Answer from the drawing. Dimensions are ordinates in mm from the lowest x, y and z of the part. Round coordinates to 2 decimals unless told otherwise and drop trailing zeros. Order: outer loops, then holes, each group sorted by start corner. A loop starts at its lowest first (then second) coordinate and runs counter-clockwise, first axis right, second up.
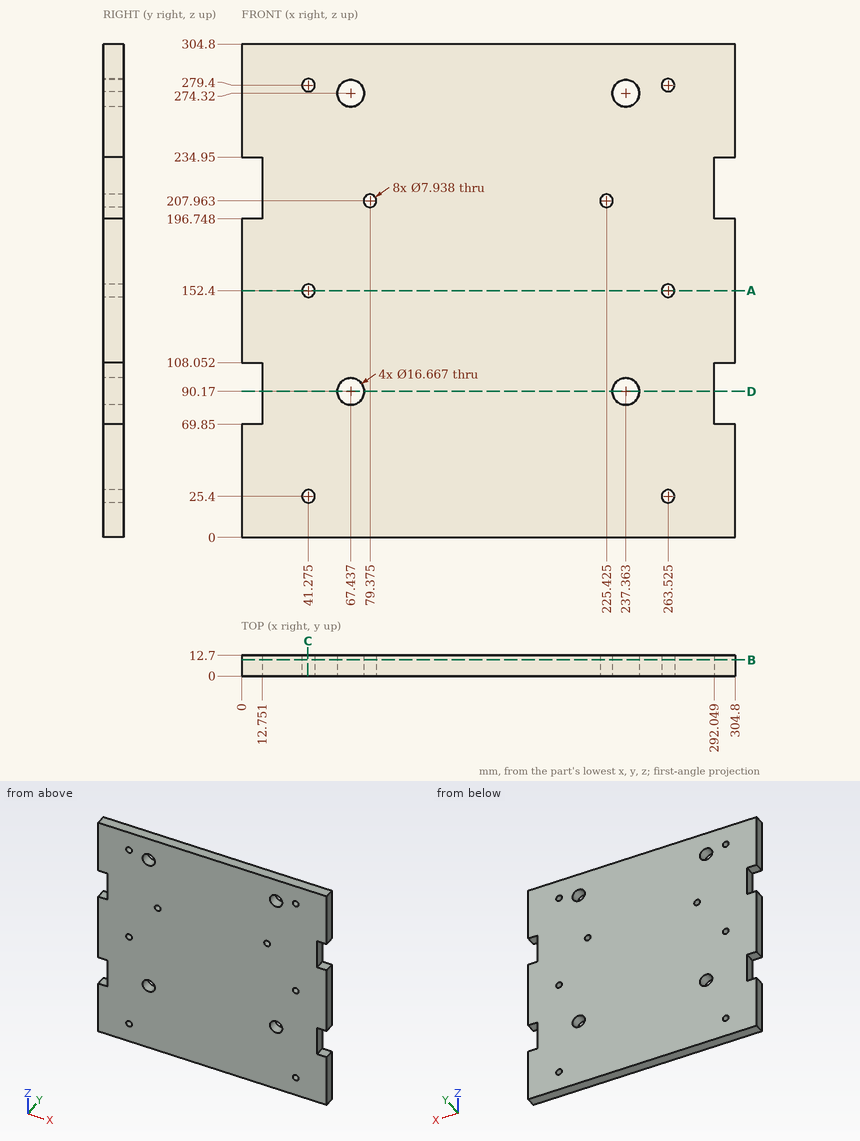
Q1. A cutting plane is placed at D-D, the plane z = 90.17. Give the vertices of the cut face in (x, y), plus the area to 3 significant figures.
Outcome:
outline: (12.75, 0) - (59.1, 0) - (59.1, 12.7) - (12.75, 12.7) - close; (75.77, 0) - (229.03, 0) - (229.03, 12.7) - (75.77, 12.7) - close; (245.7, 0) - (292.05, 0) - (292.05, 12.7) - (245.7, 12.7) - close
area: 3,120 mm2
Q2. A cutting plane is placed at A-A, the plane z = 152.4. Give the vertices of the cut face in (x, y).
Outcome:
outline: (0, 0) - (37.31, 0) - (37.31, 12.7) - (0, 12.7) - close; (45.24, 0) - (259.56, 0) - (259.56, 12.7) - (45.24, 12.7) - close; (267.49, 0) - (304.8, 0) - (304.8, 12.7) - (267.49, 12.7) - close
Q3. A cutting plane is placed at B-B, the plane y = 10. Give the number of separate pieces and of enclosed holes in the cut face, plus the area to 3 significant figures.
Outcome:
separate pieces: 1
enclosed holes: 12
area: 89,700 mm2
Q4. A cutting plane is placed at C-C, the plane x = 41. Give the vertices of the cut face in (y, z), plus the area to 3 significant figures.
Outcome:
outline: (0, 0) - (12.7, 0) - (12.7, 21.44) - (0, 21.44) - close; (0, 29.36) - (12.7, 29.36) - (12.7, 148.44) - (0, 148.44) - close; (0, 156.36) - (12.7, 156.36) - (12.7, 275.44) - (0, 275.44) - close; (0, 283.36) - (12.7, 283.36) - (12.7, 304.8) - (0, 304.8) - close
area: 3,570 mm2
Q5. Flat-ended cylindrical pins translate along their axes: pin 1 (2 mm diameter, centred on y = 11, z = 231.5, fed in from +X); pin 2 (6.5 mm diameter, centred on y = 9, z = 223.5, fed in from -X). Find the tip coordinate at first contact, or state that the pin passes through.
Outcome:
pin 1: stops at x = 292.05
pin 2: stops at x = 12.75
Q6. Straight lines are drawn through the part: probe 1 along X at (y, z) = (7.75, 90.17); probe 2 along X at (y, z) = (10.25, 279.4) (1 decimal); probe 3 along Z at (x, y) = (243, 1). For each, find the intervals that lie inside material, in ascending order.
Outcome:
probe 1: x = 12.75 to 59.1, 75.77 to 229.03, 245.7 to 292.05
probe 2: x = 0 to 37.3, 45.2 to 60.8, 74 to 230.8, 244 to 259.6, 267.5 to 304.8
probe 3: z = 0 to 84.03, 96.31 to 268.18, 280.46 to 304.8
